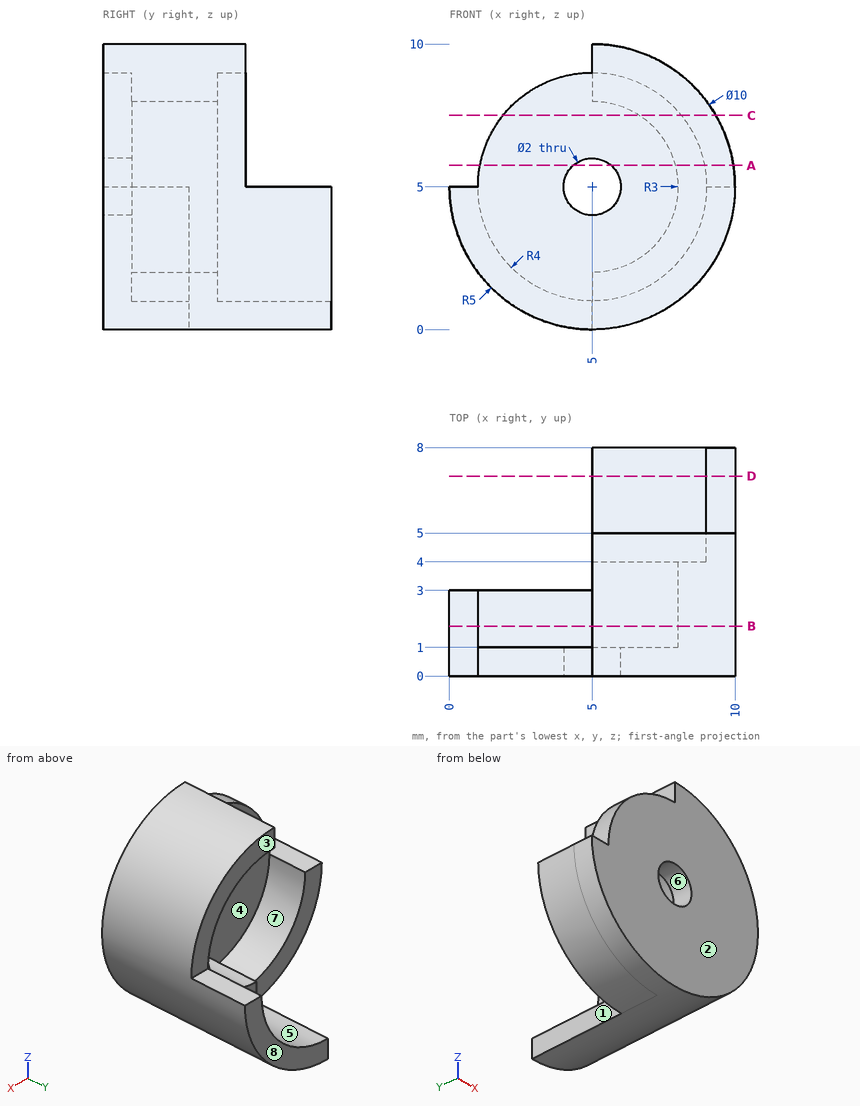
Can you work these out from the drawing? Everything is in mm from the part's minimum corner. A direction names the side the tool comes from. Give positions to 0.01 mm unless a question says otherwise; leave off trailing zeros. Order: outer loops, then holes, each group sorted by start corner. A loop starts at its lowest first (then second) coordinate and runs counter-clockwise, first axis right, second up.
1. We'd pull the mould along Z, two halves only. Please class the marked faces 6, 7 and 8: pulls with the +Z half, pulls with the -Z half, needs draft (parallel to the pull), parting line crosses it, or undercut.
2. Suppose I cut it at C-C (z = 7.5). List the corners of the cut face in (x, y) for me, plus the area to 3 significant figures.
3. Suppose I cut it at A-A (z = 5.75). List the corners of the cut face in (x, y) for me.
4. I need wall thicknesses on L1, parallel to Y at x = 4.5, z = 0.5; L2, parallel to Y at x = 8.5, z = 6; L3, parallel to Z at x = 8, y = 4.25. Which ranges of each line are inside material? Lowest first, please.
5. Will these pins go through, and if not, where does the flat tip stop? P1, Ø3, axis at x = 6.5, z = 8.5, coming from the +Y side; P2, Ø1, axis at y = 2, z = 9, coming from the -X side; P3, Ø2, axis at y = 3.5, z = 1, coming from the -X side; P4, Ø1.6, axis at x = 5, z = 5, coming from the -Y side.
6. Suppose I cut it at B-B (y = 1.75). List the corners of the cut face in (x, z) for me.
7. For the marked faces 1, 2, 3, 4 and 5, which set-ups out of +Z, -Z, +X, -X, +Y, -Y let a thin tool reach every point of the face, with its end or its side?
8. Suppose I cut it at D-D (y = 7). List the corners of the cut face in (x, z) for me.
Solved:
1. face 6: undercut
1. face 7: pulls with the +Z half
1. face 8: needs draft
2. outline: (1.88, 0) - (9.33, 0) - (9.33, 5) - (8.12, 5) - (8.12, 4) - (6.66, 4) - (6.66, 1) - (1.88, 1) - close
2. area: 16.7 mm2
3. outline: (1.07, 0) - (4.34, 0) - (4.34, 1) - (1.07, 1) - close; (5.66, 0) - (9.94, 0) - (9.94, 5) - (8.93, 5) - (8.93, 4) - (7.9, 4) - (7.9, 1) - (5.66, 1) - close
4. L1: y = 0 to 3
4. L2: y = 0 to 4
4. L3: z = 1 to 2.35, 7.65 to 9
5. P1: stops at y = 5
5. P2: stops at x = 5
5. P3: stops at x = 1.1
5. P4: passes through
6. outline: (0, 5) arc R5 ccw (long way) to (5, 10) - (5, 8) arc R3 cw to (5, 2) - (5, 1) arc R4 cw to (1, 5) - close
7. face 1: +Z, +Y
7. face 2: +Z, -Z, +X, -X, -Y
7. face 3: +Z, +X, -X, +Y
7. face 4: +Y
7. face 5: -X, +Y
8. outline: (5, 0) arc R5 ccw to (10, 5) - (9, 5) arc R4 cw to (5, 1) - close
